```python
from build123d import *

# Parameters (mm, degrees)
BASE_EXTRUSION_DEPTH    = 8
BOSS_EXTRU_1_DEPTH      = 3
ESQUISSE4_R             = 6
ENL_V_MAT_EXTRU_1_DEPTH = 34.262346156
ESQUISSE5_R             = 5
ENL_V_MAT_EXTRU_2_DEPTH = 6.5
BOSS_EXTRU_2_START      = 1
ESQUISSE6_R             = 6.5
ESQUISSE6_R_2           = 5
BOSS_EXTRU_2_DEPTH      = 1


with BuildPart() as part:
    # Esquisse1 → Base-Extrusion (new body)
    with BuildSketch(Plane.XY):
        with BuildLine():
            Line((-10.5, 13), (-10.5, -6))
            ThreePointArc((-10.5, -6), (-11.085786438, -7.414213562), (-12.5, -8))
            Line((-12.5, -8), (-19.595917942, -8))
            ThreePointArc((-19.595917942, -8), (-21.301523673, -8.955534064), (-21.377365028, -10.909090909))
            ThreePointArc((-21.377365028, -10.909090909), (0, -24), (21.377365028, -10.909090909))
            ThreePointArc((21.377365028, -10.909090909), (21.301523673, -8.955534064), (19.595917942, -8))
            Line((19.595917942, -8), (12.5, -8))
            ThreePointArc((12.5, -8), (11.085786438, -7.414213562), (10.5, -6))
            Line((10.5, -6), (10.5, 13))
            ThreePointArc((10.5, 13), (0, 23.5), (-10.5, 13))
        make_face()
    extrude(amount=BASE_EXTRUSION_DEPTH)

    # Esquisse2 → Boss.-Extru.1 (add)
    with BuildSketch(Plane.XY.offset(8)):
        with BuildLine():
            Line((-19.595917942, -8), (-11.135528726, -8))
            ThreePointArc((-11.135528726, -8), (-10.781975335, -7.968501969), (-10.43955818, -7.875))
            ThreePointArc((-10.43955818, -7.875), (0, -6), (10.43955818, -7.875))
            ThreePointArc((10.43955818, -7.875), (10.781975335, -7.968501969), (11.135528726, -8))
            Line((11.135528726, -8), (19.595917942, -8))
            ThreePointArc((19.595917942, -8), (21.301523673, -8.955534064), (21.377365028, -10.909090909))
            ThreePointArc((21.377365028, -10.909090909), (0, -24), (-21.377365028, -10.909090909))
            ThreePointArc((-21.377365028, -10.909090909), (-21.301523673, -8.955534064), (-19.595917942, -8))
        make_face()
    extrude(amount=BOSS_EXTRU_1_DEPTH)

    # Esquisse4 → Enlèv. mat.-Extru.1 (cut, through all)
    with BuildSketch(Plane.XY.offset(8)):
        with Locations((0, 13)):
            Circle(ESQUISSE4_R)
    extrude(amount=-ENL_V_MAT_EXTRU_1_DEPTH, mode=Mode.SUBTRACT)

    # Esquisse5 → Enlèv. mat.-Extru.2 (cut)
    with BuildSketch(Plane(origin=(0, 0, 0), x_dir=(-1, 0, 0), z_dir=(0, 0, -1))):
        Circle(ESQUISSE5_R)
    extrude(amount=-ENL_V_MAT_EXTRU_2_DEPTH, mode=Mode.SUBTRACT)

    # Esquisse6 → Boss.-Extru.2 (add)
    with BuildSketch(Plane(origin=(0, 0, 0), x_dir=(-1, 0, 0), z_dir=(0, 0, -1)).offset(BOSS_EXTRU_2_START)):
        with Locations(Location((0, 0, 0), (0, 0, 180))):
            Circle(ESQUISSE6_R)
        Circle(ESQUISSE6_R_2, mode=Mode.SUBTRACT)
    extrude(amount=-BOSS_EXTRU_2_DEPTH)


solid = part.part
```
The listing builds one solid part. Answer for the finished solid, in the listing's coordinates (mm). A direction names the side the tool comes from. Give positions to 0.01 mm unless a question says otherwise; leave off trailing zeros. Order: outer loops, then holes, each group sorted by start corner. A loop starts at its lowest first (then second) coordinate and runs counter-clockwise, first axis right, second up. Notation, with made-up numbers: (32, 53) - (70, 53) arc R15 cw to (70, 63) - close; hole circle Ø5 at (47, 52). An arc over 180 degrees is marked (long way). Use one line per item in the form item = value. Start each with the question number.
(1) A cutting plane is placed at B-B, the plane z = 3.5. Write down the section's boundary in (x, y), then the cut area to 3 significant figures.
(2) Consider line 1 (Y direction, x = 0, z = 2.5); line 2 (Y direction, x = -2, z = 1.5); line 3 (X direction, y = -6, z = 4.5). Determine where each line is inside the solid, lowest interval first. Write a range as from..to.
(3) Flat-ended cylindrical pins translate along their axes: pin 1 Ø6 at (x, z) = (13.5, 5.5) entering from -Y; pin 2 Ø11 at (x, y) = (1.5, -2) entering from -Z; pin 3 Ø2 at (x, z) = (-9, 5.5) entering from -Y; pin 4 Ø6.5 at (y, z) = (2, 2) entering from -X. Find the tip coordinate at first contact, or state that the pin passes through.
(4) A cutting plane is placed at D-D, the plane z = 10. Write down the section's boundary in (x, y) (3 decimals).
(5) The mould has two halves that part along Y. Classify faces 4 (the cylindrical face through (0, -6, 9)), 5 (the flat face through (10.5, 3, 4)), 6 (the flat face through (0, 0, 6.5)), 7 (the cylindrical face through (1.08, -4.88, 2.7)): released by +Y, released by -Y, zero draft, split by the parting line, or undercut.
(6) A cutting plane is placed at A-A, the plane x = 0. Write down the section's boundary in (y, z), then the cut area to 3 significant figures.
(7) For faces 1 (the flat face through (4.5, -5.2, 0)), 2 (the flat face through (2, 5, -1)), 3 (the flat face through (-10.5, 4, 4)), determine the directions among +Z, -Z, +X, -X, +Y, -Y from which every point of the face is accessible in a straight line to the end or side of a thin tool.
(8) A cutting plane is placed at C-C, the plane y = 0. Write down the section's boundary in (x, z), then the cut area to 3 significant figures.
Ans:
q1.outline = (-21.38, -10.91) arc R24 ccw to (21.38, -10.91) arc R2 ccw to (19.6, -8) - (12.5, -8) arc R2 cw to (10.5, -6) - (10.5, 13) arc R10.5 ccw to (-10.5, 13) - (-10.5, -6) arc R2 cw to (-12.5, -8) - (-19.6, -8) arc R2 ccw to start; hole circle Ø12 at (0, 13); hole circle Ø10 at (0, 0)
q1.area = 948 mm^2
q2.line_1 = -24..-5, 5..7, 19..23.5
q2.line_2 = -23.92..-4.58, 4.58..7.34, 18.66..23.31
q2.line_3 = -10.5..10.5
q3.pin_1 = -21.58
q3.pin_2 = -1
q3.pin_3 = -22.63
q3.pin_4 = -10.5
q4.outline = (-21.377, -10.909) arc R24 ccw to (21.377, -10.909) arc R2 ccw to (19.596, -8) - (11.136, -8) arc R2 cw to (10.44, -7.875) arc R30 ccw to (-10.44, -7.875) arc R2 cw to (-11.136, -8) - (-19.596, -8) arc R2 ccw to start
q5.face_4 = released by +Y
q5.face_5 = zero draft
q5.face_6 = undercut
q5.face_7 = undercut
q6.outline = (-24, 0) - (-6.5, 0) - (-6.5, -1) - (-5, -1) - (-5, 6.5) - (5, 6.5) - (5, -1) - (6.5, -1) - (6.5, 0) - (7, 0) - (7, 8) - (-6, 8) - (-6, 11) - (-24, 11) - close; (19, 0) - (23.5, 0) - (23.5, 8) - (19, 8) - close
q6.area = 276 mm^2
q7.face_1 = -Z
q7.face_2 = -Z, +X, -X, +Y, -Y
q7.face_3 = +Z, -Z, -X, +Y
q8.outline = (-10.5, 0) - (-6.5, 0) - (-6.5, -1) - (-5, -1) - (-5, 6.5) - (5, 6.5) - (5, -1) - (6.5, -1) - (6.5, 0) - (10.5, 0) - (10.5, 8) - (-10.5, 8) - close
q8.area = 106 mm^2
